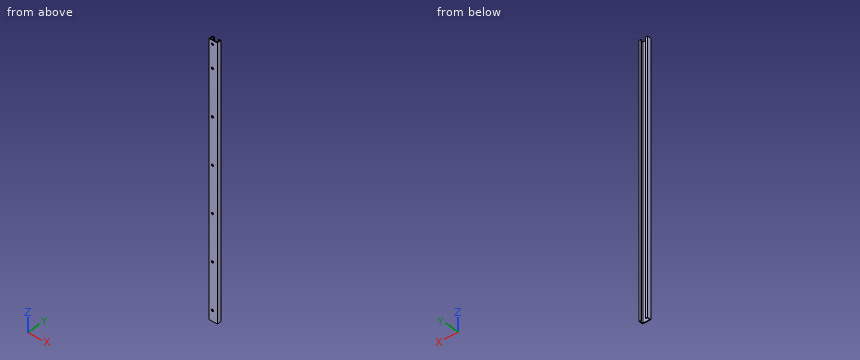
```python
from build123d import *

# Parameters (mm, degrees)
BOSS_EXTRU_1_DEPTH         = 813
D_GAGEMENT_M61_D           = 6.6
R_P_TITION_LIN_AIRE1_COUNT = 12
R_P_TITION_LIN_AIRE1_PITCH = 70


with BuildPart() as part:
    # Esquisse1 → Boss.-Extru.1 (new body)
    with BuildSketch(Plane.XY):
        Polygon((-6.5, 12.5), (-12.5, 12.5), (-12.5, 0), (12.5, 0), (12.5, 12.5), (6.5, 12.5), (6.5, 10.5), (10.5, 10.5), (10.5, 2), (-10.5, 2), (-10.5, 10.5), (-6.5, 10.5), align=None)
    extrude(amount=BOSS_EXTRU_1_DEPTH)

    # Dégagement M61 (through all)
    with Locations(Plane(origin=(0, 0, 0), x_dir=(-1, 0, 0), z_dir=(0, -1, 0))):
        with Locations((2.40627347, -801.806864395)):
            d_gagement_m61 = Hole(D_GAGEMENT_M61_D / 2)

    # Répétition linéaire1: Dégagement M61 ×12, 5 skipped
    with Locations(*[(0, 0, -i * R_P_TITION_LIN_AIRE1_PITCH) for i in range(1, R_P_TITION_LIN_AIRE1_COUNT) if i not in (2, 4, 6, 8, 10)]):
        add(d_gagement_m61, mode=Mode.SUBTRACT)


solid = part.part
```
Can you work these out from the model? Positions are in its coordinate system, mm. Give positions to 0.01 mm unless a question says otherwise; leave off trailing zeros. Loops run counter-clockwise (first coordinate to the right, second up) from the corner with the lowest first, then second, coordinate; pieces in that order, holes last. Notation, with made-up numbers: M 83.25,-31.75 L 107.25,-31.75 A16 cw 107.25,-13.75 Z; hole C 7,39.25 d6. An arc over 180 degrees is marked long. Answer in a Markdown table with one row per item.
1. For pin 1 Ø6.5 at (x, z) = (-3, 325.5) entering from +Y, with a flat end and sliding along its axis, tell me the tip position at first contact or that it passes through.
Taken from the geometry:
| item | result |
|---|---|
| pin 1 | stops at y = 2 |
2. If I drill on line 1 along X through (y, z) = (11.75, 623.5); line 2 along X through (y, z) = (2.5, 299.5); line 3 along Y through (x, z) = (-10, 602.5), over which ranges is the centre line in solid material (lowest first)?
Taken from the geometry:
| item | result |
|---|---|
| line 1 | x = -12.5 to -6.5, 6.5 to 12.5 |
| line 2 | x = -12.5 to -10.5, 10.5 to 12.5 |
| line 3 | y = 0 to 2, 10.5 to 12.5 |
3. Suppose I cut it at A-A on y = 5. Write out the boundary of the cut face in (x, z).
Taken from the geometry:
| item | result |
|---|---|
| outline | M -12.5,0 L -10.5,0 L -10.5,813 L -12.5,813 Z; M 10.5,0 L 12.5,0 L 12.5,813 L 10.5,813 Z |
4. Suppose I cut it at B-B on z = 51.5. Write out the boundary of the cut face in (x, y), plus the area to 3 significant figures.
Taken from the geometry:
| item | result |
|---|---|
| outline | M -12.5,0 L 12.5,0 L 12.5,12.5 L 6.5,12.5 L 6.5,10.5 L 10.5,10.5 L 10.5,2 L -10.5,2 L -10.5,10.5 L -6.5,10.5 L -6.5,12.5 L -12.5,12.5 Z |
| area | 108 mm² |
